Work out the finished part from the listing and answer in its coordinate system (mm). A direction names the side the tool comes from. Round coordinates to 2 decimals unless told otherwise and drop trailing zeros. Order: outer loops, then holes, each group sorted by start corner. A loop starts at its lowest first (then second) coordinate and runs counter-clockwise, first axis right, second up. Notation, with made-up numbers: (80, 82) - (91, 82) arc R20 cw to (91, 103) - close; hole circle Ø11 at (64, 9.25). An arc over 180 degrees is marked (long way). Answer in a Markdown table with one row per item.
from build123d import *

# Parameters (mm, degrees)
SKETCH1_R           = 1.9
SKETCH1_R_2         = 1.2
BOSS_EXTRUDE1_DEPTH = 3.5
SKETCH2_R           = 5.9
SKETCH2_R_2         = 4.9
BOSS_EXTRUDE2_DEPTH = 1.5
BOSS_EXTRUDE3_DEPTH = 0.25
CIRPATTERN1_COUNT   = 3


with BuildPart() as part:
    # Sketch1 → Boss-Extrude1 (new body)
    with BuildSketch(Plane.XY):
        Circle(SKETCH1_R)
        Circle(SKETCH1_R_2, mode=Mode.SUBTRACT)
    extrude(amount=BOSS_EXTRUDE1_DEPTH)



with BuildPart() as body_2:
    # Sketch2 → Boss-Extrude2 (new body)
    with BuildSketch(Plane.XY):
        Circle(SKETCH2_R)
        Circle(SKETCH2_R_2, mode=Mode.SUBTRACT)
    extrude(amount=BOSS_EXTRUDE2_DEPTH)


with BuildPart() as part_1:
    add(part.part)

    add(body_2.part)  # Boss-Extrude3 merges body 2
    # Sketch3 → Boss-Extrude3 (add, symmetric)
    with BuildSketch(Plane(origin=(0, 0, 0), x_dir=(0, 0, -1), z_dir=(1, 0, 0))):
        Polygon((0, 4.9), (-1.5, 4.9), (-3.5, 1.885172848), (-3.5, 1.643172848), (0, 1.643172848), align=None)
    boss_extrude3 = extrude(amount=BOSS_EXTRUDE3_DEPTH, both=True)

    # CirPattern1: Boss-Extrude3 ×3 about axis
    cirpattern1_axis = Axis((0, 0, 0), (0, 0, 1))
    for i in range(1, CIRPATTERN1_COUNT):
        add(boss_extrude3.rotate(cirpattern1_axis, i * 360 / CIRPATTERN1_COUNT))


solid = part_1.part
1) Find section C-C, the plane y = 4.75. Give the vertices of the cut face in (x, z).
Filled in:
| item | result |
|---|---|
| outline | (-3.5, 0) - (-1.2, 0) - (-1.2, 1.5) - (-3.5, 1.5) - close; (-0.25, 0) - (0.25, 0) - (0.25, 1.6) - (-0.25, 1.6) - close; (1.2, 0) - (3.5, 0) - (3.5, 1.5) - (1.2, 1.5) - close |
2) Each of these flat-tipped pins is pushed along its axis until it touches: pin 1 (1.5 mm diameter, centred on y = -4.5, z = 0.5, fed in from -X); pin 2 (2 mm diameter, centred on x = -2, z = 3, fed in from -Y). Where does it stop, or does it pass through?
Filled in:
| item | result |
|---|---|
| pin 1 | stops at x = -4.55 |
| pin 2 | stops at y = -1.93 |
3) Find the intervals of material crossed by probe 1 along Y at (x, z) = (1, 0.7); probe 2 along X at (y, z) = (2.5, 0.8); probe 3 along Y at (x, z) = (-2, 0.35), in increasing order. Write a range as from..to.
Filled in:
| item | result |
|---|---|
| probe 1 | y = -5.81..-4.8, -1.62..-0.66, 0.66..1.62, 4.8..5.81 |
| probe 2 | x = -5.34..-4.21, -0.25..0.25, 4.21..5.34 |
| probe 3 | y = -5.55..-4.47, -1.44..-0.87, 4.47..5.55 |
4) Find section D-D, the plane z = 0.55. Give the vertices of the cut face in (x, y).
Filled in:
| item | result |
|---|---|
| outline | circle Ø11.8 at (0, 0); hole (-4.36, -2.23) - (-1.76, -0.73) arc R1.9 cw to (-0.25, 1.88) - (-0.25, 4.89) arc R4.9 ccw to start; hole (-4.11, -2.66) arc R4.9 ccw to (4.11, -2.66) - (1.51, -1.16) arc R1.9 cw to (-1.51, -1.16) - close; hole circle Ø2.4 at (0, 0); hole (0.25, 1.88) arc R1.9 cw to (1.76, -0.73) - (4.36, -2.23) arc R4.9 ccw to (0.25, 4.89) - close |
5) Find section A-A, the plane x = 0. Give the number of separate pieces and of enclosed holes in the cut face, then the cut area to 3 significant figures.
Filled in:
| item | result |
|---|---|
| separate pieces | 3 |
| enclosed holes | 0 |
| area | 15.4 mm^2 |
6) The mould has two halves that part along Y. Classify faces 1 (the face through (-5.894, 0.259, 0.74)), 2 (the face through (-2.79, -1.32, 1.39)), 3 (the face through (1, 5, 1.5)): released by +Y, released by -Y, zero draft, split by the parting line, or undercut.
Filled in:
| item | result |
|---|---|
| face 1 | split by the parting line |
| face 2 | undercut |
| face 3 | zero draft |
7) Find section B-B, the plane y = 0. Give the vertices of the cut face in (x, z).
Filled in:
| item | result |
|---|---|
| outline | (-5.9, 0) - (-4.9, 0) - (-4.9, 1.5) - (-5.9, 1.5) - close; (-1.9, 0) - (-1.2, 0) - (-1.2, 3.5) - (-1.9, 3.5) - close; (1.2, 0) - (1.9, 0) - (1.9, 3.5) - (1.2, 3.5) - close; (4.9, 0) - (5.9, 0) - (5.9, 1.5) - (4.9, 1.5) - close |
8) Which of the six approach directions +Z, -Z, +X, -X, +Y, -Y give full straight-line access (tool end or side, diameter ignored) to faces 4 (the face through (-0.25, 3, 1)), 5 (the face through (2.95, -1.71, 2.49))?
Filled in:
| item | result |
|---|---|
| face 4 | +Z, -Z |
| face 5 | +Z, +X, -Y |
